from build123d import *

# Parameters (mm, degrees)
SKETCH1_W               = 81
SKETCH1_H               = 76
SKETCH1_W_2             = 17
SKETCH1_H_2             = 70
SKETCH1_W_3             = 15
BOSS_EXTRUDE2_DEPTH     = 20
SKETCH3_W               = 81
SKETCH3_H               = 76
BOSS_EXTRUDE3_DEPTH     = 2
CUT_EXTRUDE2_DEPTH      = 2
SKETCH5_W               = 17
SKETCH5_H               = 70
SKETCH5_R               = 1.5
CUT_EXTRUDE3_DEPTH      = 21
CUT_EXTRUDE3_DEPTH_BACK = 3


with BuildPart() as part:
    # Sketch1 → Boss-Extrude2 (new body)
    with BuildSketch(Plane.XY):
        with Locations((40.5, -38)):
            Rectangle(SKETCH1_W, SKETCH1_H)
        with Locations((31.5, -38)):
            Rectangle(SKETCH1_W_2, SKETCH1_H_2, mode=Mode.SUBTRACT)
        with Locations((11.5, -38)):
            Rectangle(SKETCH1_W_2, SKETCH1_H_2, mode=Mode.SUBTRACT)
        with Locations((50.5, -38)):
            Rectangle(SKETCH1_W_3, SKETCH1_H_2, mode=Mode.SUBTRACT)
        with Locations((69.5, -38)):
            Rectangle(SKETCH1_W_2, SKETCH1_H_2, mode=Mode.SUBTRACT)
    extrude(amount=BOSS_EXTRUDE2_DEPTH)

    # Sketch3 → Boss-Extrude3 (add)
    with BuildSketch(Plane.XY.offset(20)):
        with Locations((40.5, -38)):
            Rectangle(SKETCH3_W, SKETCH3_H)
    extrude(amount=BOSS_EXTRUDE3_DEPTH)

    # Sketch4 → Cut-Extrude2 (cut)
    with BuildSketch(Plane(origin=(0, 0, 20), x_dir=(-1, 0, 0), z_dir=(0, 0, -1))):
        with BuildLine():
            ThreePointArc((-13, -38), (-11.5, -39.5), (-10, -38))
            Line((-10, -38), (-13, -38))
        make_face()
        with BuildLine():
            Line((-13, -38), (-10, -38))
            ThreePointArc((-10, -38), (-11.5, -36.5), (-13, -38))
        make_face()
        with BuildLine():
            ThreePointArc((-33, -38), (-31.5, -39.5), (-30, -38))
            Line((-30, -38), (-33, -38))
        make_face()
        with BuildLine():
            Line((-33, -38), (-30, -38))
            ThreePointArc((-30, -38), (-31.5, -36.5), (-33, -38))
        make_face()
        with BuildLine():
            ThreePointArc((-52, -38), (-50.5, -39.5), (-49, -38))
            Line((-49, -38), (-52, -38))
        make_face()
        with BuildLine():
            Line((-52, -38), (-49, -38))
            ThreePointArc((-49, -38), (-50.5, -36.5), (-52, -38))
        make_face()
        with BuildLine():
            ThreePointArc((-71, -38), (-69.5, -39.5), (-68, -38))
            Line((-68, -38), (-71, -38))
        make_face()
        with BuildLine():
            Line((-71, -38), (-68, -38))
            ThreePointArc((-68, -38), (-69.5, -36.5), (-71, -38))
        make_face()
    extrude(amount=-CUT_EXTRUDE2_DEPTH, mode=Mode.SUBTRACT)

    # Sketch5 → Cut-Extrude3 (cut, two sides)
    with BuildSketch(Plane(origin=(0, 0, 20), x_dir=(-1, 0, 0), z_dir=(0, 0, -1))) as cut_extrude3_sk:
        Polygon((-61, 3.586024283), (-61, -3), (-78, -3), (-78, -73), (-61, -73), (-61, -79.125259563), (-89.801346659, -78.428276056), (-91.298539163, 3.586024283), align=None)
        with Locations((-69.5, -38)):
            Rectangle(SKETCH5_W, SKETCH5_H)
        with Locations((-69.5, -38)):
            Circle(SKETCH5_R, mode=Mode.SUBTRACT)
    extrude(amount=CUT_EXTRUDE3_DEPTH, mode=Mode.SUBTRACT)
    extrude(cut_extrude3_sk.sketch, amount=-CUT_EXTRUDE3_DEPTH_BACK, mode=Mode.SUBTRACT)


solid = part.part
Can you work these out from the model? Positions are in its coordinate system, mm. A direction names the side the tool comes from. Give positions to 0.01 mm unless a question says otherwise; leave off trailing zeros. Order: outer loops, then holes, each group sorted by start corner. A loop starts at its lowest first (then second) coordinate and runs counter-clockwise, first axis right, second up. Notation, with made-up numbers: M 65,29.5 L 87,29.5 A15 cw 87,58.5 Z; hole C 0.25,2.5 d5. An arc over 180 degrees is marked long. One line per question, with ' | ' between items.
Item 1: Suppose I cut it at C-C, the plane z = 10.25. Write out the boundary of the cut face in (x, y).
Answer block:
outline: M 0,-76 L 61,-76 L 61,0 L 0,0 Z; hole M 3,-73 L 20,-73 L 20,-3 L 3,-3 Z; hole M 23,-73 L 40,-73 L 40,-3 L 23,-3 Z; hole M 43,-73 L 58,-73 L 58,-3 L 43,-3 Z
Item 2: Suppose I cut it at B-B, the plane y = -38. Write out the boundary of the cut face in (x, z), then the cut area to 3 significant figures.
Answer block:
outline: M 0,0 L 3,0 L 3,20 L 10,20 L 10,22 L 0,22 Z; M 13,20 L 20,20 L 20,0 L 23,0 L 23,20 L 30,20 L 30,22 L 13,22 Z; M 33,20 L 40,20 L 40,0 L 43,0 L 43,20 L 49,20 L 49,22 L 33,22 Z; M 52,20 L 58,20 L 58,0 L 61,0 L 61,22 L 52,22 Z | area: 344 mm2
Item 3: For faces 5 (the face through (11, -3, 10)), 6 (the face through (0, -39, 11)), which set-ups out of +Z, -Z, +X, -X, +Y, -Y let a thin tool reach every point of the face, with its end or its side?
Answer block:
face 5: -Z | face 6: +Z, -Z, -X, +Y, -Y
Item 4: Suppose I cut it at D-D, the plane x = 4. Write out the boundary of the cut face in (y, z).
Answer block:
outline: M -76,0 L -73,0 L -73,20 L -3,20 L -3,0 L 0,0 L 0,22 L -76,22 Z
Item 5: We'd pull the mould along Y, two halves only. Please class faces 1 (the face through (30, -76, 11)), 2 (the face through (3, -38, 10)), 3 (the face through (30, -37, 22)), 4 (the face through (30, 0, 11)): released by +Y, released by -Y, zero draft, split by the parting line, or undercut.
Answer block:
face 1: released by -Y | face 2: undercut | face 3: zero draft | face 4: released by +Y
Item 6: I'm going to push flat-ended pins straight in: pin 1 Ø10 at (y, z) = (-34.5, 12) entering from -X; pin 2 Ø5 at (x, y) = (8, -20.5) entering from -Z. Where does each tip first touch, or does it pass through?
Answer block:
pin 1: stops at x = 0 | pin 2: stops at z = 20
Item 7: Suppose I cut it at A-A, the plane x = 31.5. Write out the boundary of the cut face in (y, z), then the cut area to 3 significant figures.
Answer block:
outline: M -76,0 L -73,0 L -73,20 L -39.5,20 L -39.5,22 L -76,22 Z; M -36.5,20 L -3,20 L -3,0 L 0,0 L 0,22 L -36.5,22 Z | area: 266 mm2
Item 8: Please list where these lines run through material, in increasing order: L1, parallel to X at y = -13, z = 13.75; L2, parallel to Y at x = 31.5, z = 20.4; L3, parallel to Y at x = 46.5, z = 13.5.
Answer block:
L1: x = 0 to 3, 20 to 23, 40 to 43, 58 to 61 | L2: y = -76 to -39.5, -36.5 to 0 | L3: y = -76 to -73, -3 to 0
